For this review, take the finished solid that the model builds, in its own axes (mm). Coordinates: 2 decimals unless noted, no trailing zeros. Order: outer loops, then holes, each group sorted by start corner. A loop starts at its lowest first (then second) coordinate and runs counter-clockwise, first axis right, second up. Notation, with made-up numbers: (64, -23.75) -> (99, -23.75) arc R26 cw to (99, 8.25) -> close; hole circle Ø4 at (61, 2). An arc over 180 degrees is marked (long way). Write item = value, one per line. Start each with the question number.
1) Consider section B-B on y = 8. Give the boundary of the cut face in (x, z) (1 decimal).
2) Wall thickness on probe 1 along X at (y, z) = (1.35, 129.88) (3 decimals); probe 2 along X at (y, z) = (9.5, -29) (1 decimal); probe 3 along Y at (x, z) = (4, -16): over which ranges is each line inside the solid? List them lowest first. Write a range as [from, to].
3) Insertion check: pin 1 Ø3 at (x, z) = (-2.5, -56) entering from +Y; pin 2 Ø5 at (y, z) = (6.5, -63) entering from -X; pin 3 Ø4 at (y, z) = (13.59, 50) entering from +X. Each pin has a flat end and moves straight along its axis. Give the tip position at first contact, or say it passes through.
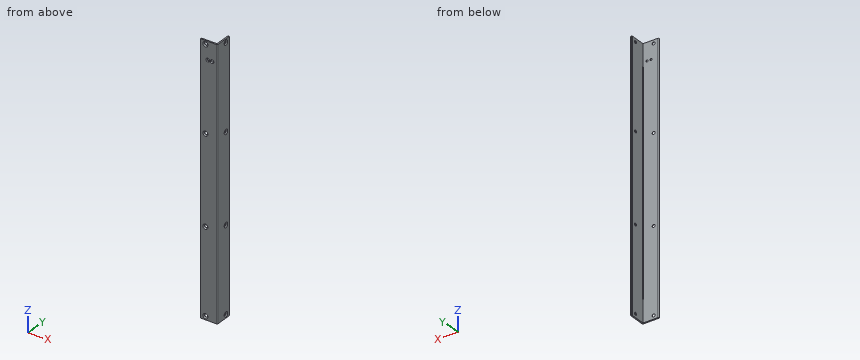
from build123d import *

# Parameters (mm, degrees)
BOSS_EXTRUDE1_DEPTH                               = 150
CSK_FOR_4_FLAT_HEAD_MACHINE_SCREW_100_D           = 3.2639
CSK_FOR_4_FLAT_HEAD_MACHINE_SCREW_100_CSINK_D     = 5.715
CSK_FOR_4_FLAT_HEAD_MACHINE_SCREW_100_CSINK_ANGLE = 100
CSK_FOR_4_FLAT_HEAD_MACHINE_SCREW_2_D             = 3.2639
CSK_FOR_4_FLAT_HEAD_MACHINE_SCREW_2_CSINK_D       = 5.715
CSK_FOR_4_FLAT_HEAD_MACHINE_SCREW_2_CSINK_ANGLE   = 100
FILLET1_R                                         = 1
F_2_CLEARANCE_HOLE1_AT_2_COUNT                    = 2
F_2_CLEARANCE_HOLE1_AT_2_PITCH                    = 4.8
CSK_FOR_4_FLAT_HEAD_MACHINE_SCREW_3_D             = 3.2639
CSK_FOR_4_FLAT_HEAD_MACHINE_SCREW_3_CSINK_D       = 5.715
CSK_FOR_4_FLAT_HEAD_MACHINE_SCREW_3_CSINK_ANGLE   = 100
CSK_FOR_4_FLAT_HEAD_MACHINE_SCREW_4_D             = 3.2639
CSK_FOR_4_FLAT_HEAD_MACHINE_SCREW_4_CSINK_D       = 5.715
CSK_FOR_4_FLAT_HEAD_MACHINE_SCREW_4_CSINK_ANGLE   = 100
CSK_FOR_4_FLAT_HEAD_MACHINE_SCREW_5_D             = 3.2639
CSK_FOR_4_FLAT_HEAD_MACHINE_SCREW_5_CSINK_D       = 5.715
CSK_FOR_4_FLAT_HEAD_MACHINE_SCREW_5_CSINK_ANGLE   = 100
CSK_FOR_4_FLAT_HEAD_MACHINE_SCREW_6_D             = 3.2639
CSK_FOR_4_FLAT_HEAD_MACHINE_SCREW_6_CSINK_D       = 5.715
CSK_FOR_4_FLAT_HEAD_MACHINE_SCREW_6_CSINK_ANGLE   = 100
CUT_EXTRUDE1_DEPTH                                = 25


with BuildPart() as part:
    # Sketch2 → Boss-Extrude1 (new, symmetric)
    with BuildSketch(Plane.XY):
        with BuildLine():
            Line((-9.525, 0), (9.525, 0))
            Line((9.525, 0), (9.525, 19.05))
            Line((9.525, 19.05), (8.73125, 19.05))
            ThreePointArc((8.73125, 19.05), (8.169983992, 18.817516008), (7.9375, 18.25625))
            Line((7.9375, 18.25625), (7.9375, 2.38125))
            ThreePointArc((7.9375, 2.38125), (7.705016008, 1.819983992), (7.14375, 1.5875))
            Line((7.14375, 1.5875), (-8.73125, 1.5875))
            ThreePointArc((-8.73125, 1.5875), (-9.292516008, 1.355016008), (-9.525, 0.79375))
            Line((-9.525, 0.79375), (-9.525, 0))
        make_face()
    extrude(amount=BOSS_EXTRUDE1_DEPTH, both=True)

    # CSK for _4 Flat Head Machine Screw _100 (through all)
    with Locations(Plane(origin=(0, 0, 0), x_dir=(-1, 0, 0), z_dir=(0, -1, 0))):
        with Locations((4.0625, -146), (4.0625, 146)):
            CounterSinkHole(CSK_FOR_4_FLAT_HEAD_MACHINE_SCREW_100_D / 2, CSK_FOR_4_FLAT_HEAD_MACHINE_SCREW_100_CSINK_D / 2, counter_sink_angle=CSK_FOR_4_FLAT_HEAD_MACHINE_SCREW_100_CSINK_ANGLE)

    # CSK for _4 Flat Head Machine Screw _ 2 (through all)
    with Locations(Plane(origin=(9.525, 0, 0), x_dir=(0, 0, -1), z_dir=(1, 0, 0))):
        with Locations((-146, 13.5875), (146, 13.5875)):
            CounterSinkHole(CSK_FOR_4_FLAT_HEAD_MACHINE_SCREW_2_D / 2, CSK_FOR_4_FLAT_HEAD_MACHINE_SCREW_2_CSINK_D / 2, counter_sink_angle=CSK_FOR_4_FLAT_HEAD_MACHINE_SCREW_2_CSINK_ANGLE)

    # Fillet1
    fillet1_edges = [part.edges().sort_by_distance(p)[0] for p in [
        (9.525, 0, 0),
    ]]
    fillet(fillet1_edges, radius=FILLET1_R)

    # Sketch30 → #2 Clearance Hole1 (revolve, cut)
    with BuildSketch(Plane(origin=(3.49375, 1.5875, 129.88), x_dir=(0, 0, 1), z_dir=(1, 0, 0))):
        Polygon((0, 0), (0, 1.5875), (2.0574, 1.5875), (1.2192, 0.623261201), (1.2192, 0), align=None)
    f_2_clearance_hole1 = revolve(axis=Axis((3.49375, 7.9375, 129.88), (0, -1, 0)), mode=Mode.SUBTRACT)

    # #2 Clearance Hole1 at 2: #2 Clearance Hole1 ×2
    with Locations(*[(-i * F_2_CLEARANCE_HOLE1_AT_2_PITCH, 0, 0) for i in range(1, F_2_CLEARANCE_HOLE1_AT_2_COUNT)]):
        add(f_2_clearance_hole1, mode=Mode.SUBTRACT)

    # CSK for _4 Flat Head Machine Screw _ 3 (through all)
    with Locations(Plane(origin=(0, 0, 0), x_dir=(-1, 0, 0), z_dir=(0, -1, 0))):
        with Locations((4.0625, 50)):
            CounterSinkHole(CSK_FOR_4_FLAT_HEAD_MACHINE_SCREW_3_D / 2, CSK_FOR_4_FLAT_HEAD_MACHINE_SCREW_3_CSINK_D / 2, counter_sink_angle=CSK_FOR_4_FLAT_HEAD_MACHINE_SCREW_3_CSINK_ANGLE)

    # CSK for _4 Flat Head Machine Screw _ 4 (through all)
    with Locations(Plane(origin=(9.525, 0, 0), x_dir=(0, 0, -1), z_dir=(1, 0, 0))):
        with Locations((50, 13.5875)):
            CounterSinkHole(CSK_FOR_4_FLAT_HEAD_MACHINE_SCREW_4_D / 2, CSK_FOR_4_FLAT_HEAD_MACHINE_SCREW_4_CSINK_D / 2, counter_sink_angle=CSK_FOR_4_FLAT_HEAD_MACHINE_SCREW_4_CSINK_ANGLE)

    # CSK for _4 Flat Head Machine Screw _ 5 (through all)
    with Locations(Plane(origin=(9.525, 0, 0), x_dir=(0, 0, -1), z_dir=(1, 0, 0))):
        with Locations((-50, 13.5875)):
            CounterSinkHole(CSK_FOR_4_FLAT_HEAD_MACHINE_SCREW_5_D / 2, CSK_FOR_4_FLAT_HEAD_MACHINE_SCREW_5_CSINK_D / 2, counter_sink_angle=CSK_FOR_4_FLAT_HEAD_MACHINE_SCREW_5_CSINK_ANGLE)

    # CSK for _4 Flat Head Machine Screw _ 6 (through all)
    with Locations(Plane(origin=(0, 0, 0), x_dir=(-1, 0, 0), z_dir=(0, -1, 0))):
        with Locations((4.0625, -50)):
            CounterSinkHole(CSK_FOR_4_FLAT_HEAD_MACHINE_SCREW_6_D / 2, CSK_FOR_4_FLAT_HEAD_MACHINE_SCREW_6_CSINK_D / 2, counter_sink_angle=CSK_FOR_4_FLAT_HEAD_MACHINE_SCREW_6_CSINK_ANGLE)

    # Sketch44 → Cut-Extrude1 (cut)
    with BuildSketch(Plane.XY.offset(150)):
        Polygon((7.9375, 6.5875), (7.9375, 1.5875), (2.9375, 1.5875), align=None)
    cut_extrude1 = extrude(amount=-CUT_EXTRUDE1_DEPTH, mode=Mode.SUBTRACT)

    # Mirror1: Cut-Extrude1 across plane
    add(cut_extrude1.mirror(Plane.XY), mode=Mode.SUBTRACT)


solid = part.part
Answer sheet:
q1.outline = (7.9, -150) -> (9.5, -150) -> (9.5, 150) -> (7.9, 150) -> close
q2.probe_1 = [-9.297, -2.525], [-0.087, 2.275], [4.713, 9.525]
q2.probe_2 = [7.9, 9.5]
q2.probe_3 = [0, 1.59]
q3.pin_1 = 1.59
q3.pin_2 = 7.94
q3.pin_3 = 8.81
